from build123d import *

# Parameters (mm, degrees)
BOSS_EXTRUDE1_DEPTH = 15
FILLET1_R           = 0.2
FILLET2_R           = 0.5
FILLET3_R           = 0.2


with BuildPart() as part:
    # Sketch1 → Boss-Extrude1 (new body)
    with BuildSketch(Plane.XY):
        Polygon((-4.5, 5.519615242), (-4.5, 7.8988893), (-7, 7.8988893), (-7, -4.1011107), (7, -4.1011107), (7, 7.8988893), (4.5, 7.8988893), (4.5, 5.519615242), (5.1, 5.519615242), (5.1, -0.6), (-5.1, -0.6), (-5.1, 5.519615242), align=None)
        Polygon((-2.5, 7.8988893), (-4.5, 7.8988893), (-4.5, 5.519615242), (-4.2, 5.519615242), (-2.5, 4.538119785), align=None)
        Polygon((4.5, 7.8988893), (2.5, 7.8988893), (2.5, 4.538119785), (4.2, 5.519615242), (4.5, 5.519615242), align=None)
    extrude(amount=BOSS_EXTRUDE1_DEPTH)

    # Fillet1
    fillet1_edges = [part.edges().sort_by_distance(p)[0] for p in [
        (4.2, 5.519615242, 7.5),
        (2.5, 4.538119785, 7.5),
        (2.5, 7.8988893, 7.5),
        (7, 7.8988893, 7.5),
        (-7, 7.8988893, 7.5),
        (-2.5, 7.8988893, 7.5),
        (-2.5, 4.538119785, 7.5),
        (-4.2, 5.519615242, 7.5),
        (-5.1, 5.519615242, 7.5),
        (5.1, 5.519615242, 7.5),
    ]]
    fillet(fillet1_edges, radius=FILLET1_R)

    # Fillet2
    fillet2_edges = [part.edges().sort_by_distance(p)[0] for p in [
        (7, -4.1011107, 7.5),
        (-7, -4.1011107, 7.5),
        (-5.1, -0.6, 7.5),
        (5.1, -0.6, 7.5),
    ]]
    fillet(fillet2_edges, radius=FILLET2_R)

    # Fillet3
    fillet3_edges = [part.edges().sort_by_distance(p)[0] for p in [
        (0, -4.1011107, 0),
        (0, -4.1011107, 15),
        (0, -0.6, 0),
        (5.1, 2.609807621, 0),
        (7, 2.0488893, 0),
        (6.853553391, -3.95466409, 0),
        (-6.853553391, -3.95466409, 0),
        (7, 2.0488893, 15),
        (5.1, 2.609807621, 15),
        (0, -0.6, 15),
        (6.853553391, -3.95466409, 15),
        (-6.853553391, -3.95466409, 15),
        (-4.953553391, -0.453553391, 0),
        (-4.953553391, -0.453553391, 15),
        (4.953553391, -0.453553391, 0),
        (4.953553391, -0.453553391, 15),
        (4.576794919, 5.519615242, 0),
        (4.576794919, 5.519615242, 15),
        (3.476794919, 5.102072594, 0),
        (3.476794919, 5.102072594, 15),
        (-3.476794919, 5.102072594, 0),
        (-3.476794919, 5.102072594, 15),
        (-4.576794919, 5.519615242, 0),
        (-4.576794919, 5.519615242, 15),
        (-5.1, 2.609807621, 0),
        (-5.1, 2.609807621, 15),
        (-7, 2.0488893, 0),
        (-7, 2.0488893, 15),
        (2.5, 6.291709623, 0),
        (4.75, 7.8988893, 0),
        (-4.75, 7.8988893, 0),
        (-2.5, 6.291709623, 0),
        (2.6, 4.711324865, 0),
        (-2.6, 4.711324865, 0),
        (-2.558578644, 7.840310656, 0),
        (2.558578644, 7.840310656, 0),
        (6.941421356, 7.840310656, 0),
        (-6.941421356, 7.840310656, 0),
        (-4.75, 7.8988893, 15),
        (-2.5, 6.291709623, 15),
        (4.75, 7.8988893, 15),
        (2.5, 6.291709623, 15),
        (2.6, 4.711324865, 15),
        (-2.6, 4.711324865, 15),
        (-2.558578644, 7.840310656, 15),
        (2.558578644, 7.840310656, 15),
        (6.941421356, 7.840310656, 15),
        (-6.941421356, 7.840310656, 15),
        (5.041421356, 5.461036599, 0),
        (5.041421356, 5.461036599, 15),
        (4.201826029, 5.512800408, 0),
        (4.201826029, 5.512800408, 15),
        (-4.201826029, 5.512800408, 0),
        (-4.201826029, 5.512800408, 15),
        (-5.041421356, 5.461036599, 0),
        (-5.041421356, 5.461036599, 15),
    ]]
    fillet(fillet3_edges, radius=FILLET3_R)


solid = part.part
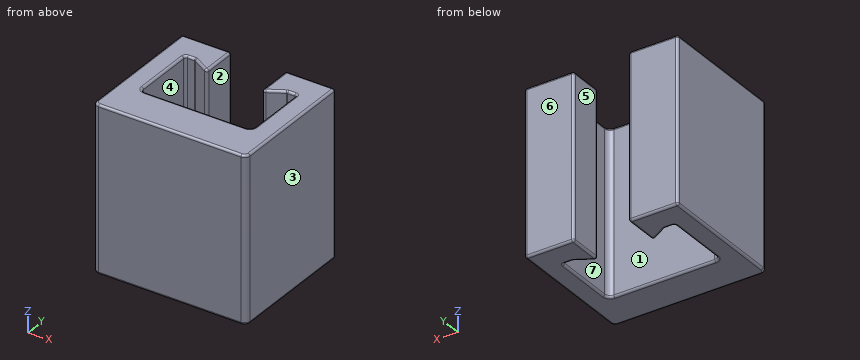
The model under review builds one solid part; all positions refer to its coordinate system, in mm. Face numbers are marked on the shaded views. A direction names the side the tool comes from. Coordinates: 2 decimals unless noted, no trailing zeros. Write each loop counter-clockwise with the first axis right and the second up, starting at its lowest first coordinate (ties: lowest second). Pieces come first, ordered by that corner, then holes. Notation, with made-up numbers: (64.5, 72.25) - (69.5, 72.25) arc R13 ccw to (69.5, 78.25) - close; hole circle Ø9 at (-14, -13.75). An arc over 180 degrees is marked (long way). Answer as CSV lines item,"result".
(1) Clearance check with a flat-ended pin moving along its axis: pin 1 Ø7.5 at (x, z) = (-1, 5.5) entering from +Y. State where the tip first meets the part, or that it passes through.
Data:
pin 1,"stops at y = 7.9"
(2) We need section B-B (z = 6.25). Give the boundary of the cut face in (x, y).
Data:
outline,"(-7, -3.6) arc R0.5 ccw to (-6.5, -4.1) - (6.5, -4.1) arc R0.5 ccw to (7, -3.6) - (7, 7.7) arc R0.2 ccw to (6.8, 7.9) - (2.7, 7.9) arc R0.2 ccw to (2.5, 7.7) - (2.5, 4.88) arc R0.2 ccw to (2.8, 4.71) - (4.15, 5.49) arc R0.2 cw to (4.25, 5.52) - (4.9, 5.52) arc R0.2 cw to (5.1, 5.32) - (5.1, -0.1) arc R0.5 cw to (4.6, -0.6) - (-4.6, -0.6) arc R0.5 cw to (-5.1, -0.1) - (-5.1, 5.32) arc R0.2 cw to (-4.9, 5.52) - (-4.25, 5.52) arc R0.2 cw to (-4.15, 5.49) - (-2.8, 4.71) arc R0.2 ccw to (-2.5, 4.88) - (-2.5, 7.7) arc R0.2 ccw to (-2.7, 7.9) - (-6.8, 7.9) arc R0.2 ccw to (-7, 7.7) - close"
(3) Mouldability with a two-part tool opening along Y and no side actions: class the marked faces 4, 5, 6 and 7 as pulls with the +Y half, pulls with the -Y half, needs draft (parallel to the pull), parting line crosses it, or undercut.
Data:
face 4,"undercut"
face 5,"needs draft"
face 6,"pulls with the +Y half"
face 7,"undercut"
(4) For line 1 along Y through (x, z) = (1.5, 12.75); line 2 along X through (y, z) = (6, 1.25); line 3 along X through (y, z) = (2, 12.5), list the stretches that pass through material, from the lowest coordinate up. Write a range as [from, to].
Data:
line 1,"y = [-4.1, -0.6]"
line 2,"x = [-7, -2.5], [2.5, 7]"
line 3,"x = [-7, -5.1], [5.1, 7]"
(5) Tool access review of the marked faces 1, 2 and 3: name each direction out of +Z, -Z, +X, -X, +Y, -Y from which nothing blocks a thin tool from reaching the whole face with its end or side.
Data:
face 1,"+Z, -Z"
face 2,"+Z, -Z, +Y"
face 3,"+Z, -Z, +X, +Y, -Y"
(6) We need section C-C (x = 1). Give the boundary of the cut face in (y, z).
Data:
outline,"(-4.1, 0.2) arc R0.2 ccw to (-3.9, 0) - (-0.8, 0) arc R0.2 ccw to (-0.6, 0.2) - (-0.6, 14.8) arc R0.2 ccw to (-0.8, 15) - (-3.9, 15) arc R0.2 ccw to (-4.1, 14.8) - close"
(7) We need section D-D (y = 7). Give the boundary of the cut face in (x, z), plus the area to 3 significant figures.
Data:
outline,"(-7, 0.2) arc R0.2 ccw to (-6.8, 0) - (-2.7, 0) arc R0.2 ccw to (-2.5, 0.2) - (-2.5, 14.8) arc R0.2 ccw to (-2.7, 15) - (-6.8, 15) arc R0.2 ccw to (-7, 14.8) - close; (2.5, 0.2) arc R0.2 ccw to (2.7, 0) - (6.8, 0) arc R0.2 ccw to (7, 0.2) - (7, 14.8) arc R0.2 ccw to (6.8, 15) - (2.7, 15) arc R0.2 ccw to (2.5, 14.8) - close"
area,"135 mm2"
(8) We need section A-A (y = 3.5). Give the boundary of the cut face in (x, z).
Data:
outline,"(-7, 0.2) arc R0.2 ccw to (-6.8, 0) - (-5.3, 0) arc R0.2 ccw to (-5.1, 0.2) - (-5.1, 14.8) arc R0.2 ccw to (-5.3, 15) - (-6.8, 15) arc R0.2 ccw to (-7, 14.8) - close; (5.1, 0.2) arc R0.2 ccw to (5.3, 0) - (6.8, 0) arc R0.2 ccw to (7, 0.2) - (7, 14.8) arc R0.2 ccw to (6.8, 15) - (5.3, 15) arc R0.2 ccw to (5.1, 14.8) - close"
